Print and shaded views of the part. All mm, measured from the part's lowest x, y and z. Round coordinates to 2 decimals unless told otherwise and drop trailing zeros. Write each loop counter-clockwise with the first axis right and the second up, starting at its lowest first coordinate (ties: lowest second). Pieces come first, ordered by that corner, then holes. Notation, with made-up numbers: M -4.75,52 L 39.25,52 A16 ccw 39.25,76 Z; hole C 80,-19.5 d3. An arc over 180 degrees is marked long. Write item = value, one per line.
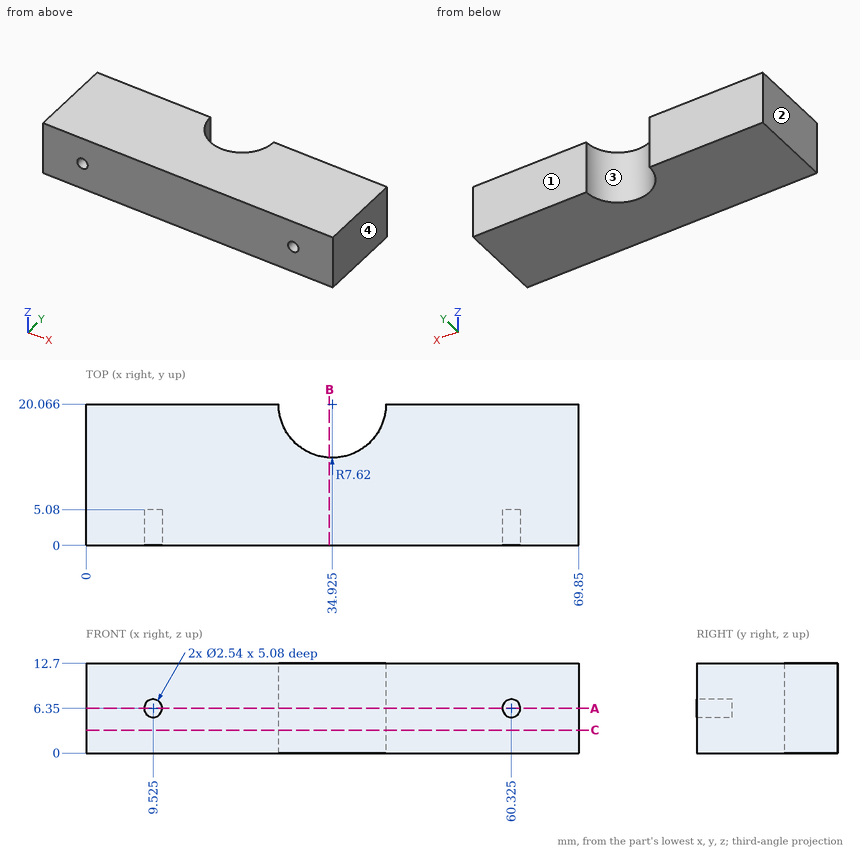
1. Band-saw the part on C-C (z = 3.25). List the corners of the cut face in (x, y) (3 decimals).
Responses:
outline = M 0,0 L 69.85,0 L 69.85,20.066 L 42.545,20.066 A7.62 cw 27.305,20.066 L 0,20.066 Z
2. Probe probe 1 along X at (y, z) = (3.3, 6.35) (3 decimals); probe 2 along X at (y, z) = (13.5, 9.5); probe 3 along Z at (x, y) = (61, 2.75). List the from-to ranges inside material, lowest first.
Responses:
probe_1 = 0 to 8.255, 10.795 to 59.055, 61.595 to 69.85
probe_2 = 0 to 31.06, 38.79 to 69.85
probe_3 = 0 to 5.27, 7.43 to 12.7
3. Band-saw the part on B-B (x = 34.5). List the corners of the cut face in (y, z), plus the area to 3 significant figures.
Responses:
outline = M 0,0 L 12.46,0 L 12.46,12.7 L 0,12.7 Z
area = 158 mm²
4. Band-saw the part on A-A (z = 6.35). List the corners of the cut face in (x, y) (3 decimals).
Responses:
outline = M 0,0 L 8.255,0 L 8.255,5.08 L 10.795,5.08 L 10.795,0 L 59.055,0 L 59.055,5.08 L 61.595,5.08 L 61.595,0 L 69.85,0 L 69.85,20.066 L 42.545,20.066 A7.62 cw 27.305,20.066 L 0,20.066 Z
5. Flat gauge pins, fed straight in: pin 1 (2 mm diameter, centred on y = 4, z = 7, fed in from -X); pin 2 (1.3 mm diameter, centred on x = 60, z = 6.5, fed in from -Y). Where does each tip first touch, or does it go through?
Responses:
pin_1 = 0
pin_2 = 5.08
6. Mould opens along X. For the marked faces 1, 2, 3 and 4 say: pulls with the +X half, pulls with the -X half, needs draft (parallel to the pull), parting line crosses it, or undercut.
Responses:
face_1 = needs draft
face_2 = pulls with the -X half
face_3 = undercut
face_4 = pulls with the +X half
